```python
from build123d import *

# Parameters (mm, degrees)
SKETCH1_W           = 26.25
SKETCH1_H           = 22
SKETCH1_R           = 3
BOSS_EXTRUDE1_DEPTH = 3
FILLET1_R           = 5
SKETCH2_R           = 1.625
CUT_EXTRUDE1_DEPTH  = 3
SKETCH5_W           = 20
SKETCH5_H           = 3
BOSS_EXTRUDE2_DEPTH = 10
SKETCH6_R           = 1.65
CUT_EXTRUDE4_DEPTH  = 28
CHAMFER1_SIZE       = 10
CHAMFER1_SIZE_2     = 17.320508076
SKETCH9_W           = 20
SKETCH9_H           = 5
CUT_EXTRUDE6_DEPTH  = 3
FILLET3_R           = 5
SKETCH16_W          = 40
SKETCH16_H          = 8
CUT_EXTRUDE11_DEPTH = 10
SKETCH17_R          = 1.25
CUT_EXTRUDE12_DEPTH = 10
SKETCH18_W          = 114.543980026
SKETCH18_H          = 4
CUT_EXTRUDE13_DEPTH = 10
SKETCH3_R           = 1.625
CUT_EXTRUDE14_DEPTH = 10


# Some blends are built 0.0001 mm under size
with BuildPart() as part:
    # Sketch1 → Boss-Extrude1 (new body)
    # profile 1 of 3: a face of its own
    with BuildSketch(Plane(origin=(0, 0, 0), x_dir=(1, 0, 0), z_dir=(0, 1, 0))):
        with Locations((18.375, 0)):
            Rectangle(SKETCH1_W, SKETCH1_H)
        with Locations(Location((20, 0, 0), (0, 0, 270))):
            Circle(SKETCH1_R, mode=Mode.SUBTRACT)
    # profile 2 of 3: a face of its own
    with BuildSketch(Plane(origin=(0, 0, 0), x_dir=(1, 0, 0), z_dir=(0, 1, 0))):
        with Locations((-18.375, 0)):
            Rectangle(SKETCH1_W, SKETCH1_H)
        with Locations(Location((-20, 0, 0), (0, 0, 270))):
            Circle(SKETCH1_R, mode=Mode.SUBTRACT)
    # profile 3 of 3: a face of its own
    with BuildSketch(Plane(origin=(0, 0, 0), x_dir=(1, 0, 0), z_dir=(0, 1, 0))):
        with BuildLine():
            Line((-5.25, -11), (-31.5, -11))
            Line((-31.5, -11), (-50, -11))
            add(Edge.make_bspline(
                [(-50, -11), (-77.2307176, -35.658609428), (-60, -76)],
                knots=[0, 0, 0, 1, 1, 1], degree=2))
            Line((-60, -76), (-22, -76))
            Line((-22, -76), (-22, -51))
            Line((-22, -51), (22, -51))
            Line((22, -51), (22, -76))
            Line((22, -76), (60, -76))
            add(Edge.make_bspline(
                [(50, -11), (77.2307176, -35.658609428), (60, -76)],
                knots=[0, 0, 0, 1, 1, 1], degree=2))
            Line((50, -11), (31.5, -11))
            Line((31.5, -11), (5.25, -11))
            Line((5.25, -11), (-5.25, -11))
        make_face()
    extrude(amount=BOSS_EXTRUDE1_DEPTH)

    # Fillet1
    fillet1_edges = [part.edges().sort_by_distance(p)[0] for p in [
        (60, 1.5, 76),
        (-60, 1.5, 76),
    ]]
    fillet(fillet1_edges, radius=FILLET1_R)

    # Sketch2 → Cut-Extrude1 (cut)
    with BuildSketch(Plane(origin=(0, 3, 0), x_dir=(1, 0, 0), z_dir=(0, 1, 0))):
        with Locations(Location((-60, -56, 0), (0, 0, 270))):
            Circle(SKETCH2_R)
        with Locations(Location((60, -56, 0), (0, 0, 270))):
            Circle(SKETCH2_R)
        with Locations(Location((-45, -17, 0), (0, 0, 270))):
            Circle(SKETCH2_R)
        with Locations(Location((-60, -34, 0), (0, 0, 270))):
            Circle(SKETCH2_R)
        with Locations(Location((60, -34, 0), (0, 0, 270))):
            Circle(SKETCH2_R)
        with Locations(Location((45, -17, 0), (0, 0, 270))):
            Circle(SKETCH2_R)
        with Locations(Location((0, -18, 0), (0, 0, 270))):
            Circle(SKETCH2_R)
        with Locations(Location((0, -36, 0), (0, 0, 270))):
            Circle(SKETCH2_R)
    extrude(amount=-CUT_EXTRUDE1_DEPTH, mode=Mode.SUBTRACT)

    # Sketch5 → Boss-Extrude2 (add)
    with BuildSketch(Plane(origin=(0, 3, 0), x_dir=(1, 0, 0), z_dir=(0, 1, 0))):
        with Locations((0, -49.5)):
            Rectangle(SKETCH5_W, SKETCH5_H)
    extrude(amount=BOSS_EXTRUDE2_DEPTH)

    # Sketch6 → Cut-Extrude4 (cut)
    with BuildSketch(Plane.XY.offset(76)):
        with Locations((0, 5)):
            Circle(SKETCH6_R)
        with Locations((0, 5.5)):
            Circle(SKETCH6_R)
        with Locations((0, 4.5)):
            Circle(SKETCH6_R)
    extrude(amount=-CUT_EXTRUDE4_DEPTH, mode=Mode.SUBTRACT)

    # Chamfer1
    # the kernel refuses this chamfer: 17.320508076, 10 mm, written as the material it adds along each edge
    with BuildSketch(Plane(origin=(-10, 3, 51), x_dir=(-0.9983227437537926, -0.05789386240267139, 0), z_dir=(0, 0, -1))) as chamfer1_piece_1_section:
        Polygon((CHAMFER1_SIZE * 0.998322743754, CHAMFER1_SIZE * 0.0578938624027), (-CHAMFER1_SIZE_2 * 0.0578938624016, CHAMFER1_SIZE_2 * 0.998322743736), (0, 0), align=None)
    chamfer1_piece_1 = extrude(amount=3, mode=Mode.PRIVATE)
    chamfer1_piece_1 = split(chamfer1_piece_1, bisect_by=Plane(origin=(-13.731694811, 13, 49.5), z_dir=(0, -1, 0)), keep=Keep.TOP, mode=Mode.PRIVATE)
    add(chamfer1_piece_1)
    with BuildSketch(Plane(origin=(10, 3, 48), x_dir=(0.9983227437537926, -0.05789386240267137, 0), z_dir=(0, 0, 1))) as chamfer1_piece_2_section:
        Polygon((CHAMFER1_SIZE * 0.998322743754, CHAMFER1_SIZE * 0.0578938624027), (-CHAMFER1_SIZE_2 * 0.0578938624016, CHAMFER1_SIZE_2 * 0.998322743736), (0, 0), align=None)
    chamfer1_piece_2 = extrude(amount=3, mode=Mode.PRIVATE)
    chamfer1_piece_2 = split(chamfer1_piece_2, bisect_by=Plane(origin=(13.731694811, 13, 49.5), z_dir=(0, -1, 0)), keep=Keep.TOP, mode=Mode.PRIVATE)
    add(chamfer1_piece_2)

    # Sketch9 → Cut-Extrude6 (cut)
    with BuildSketch(Plane(origin=(0, 3, 0), x_dir=(1, 0, 0), z_dir=(0, 1, 0))):
        with Locations((0, -45.5)):
            Rectangle(SKETCH9_W, SKETCH9_H)
    extrude(amount=-CUT_EXTRUDE6_DEPTH, mode=Mode.SUBTRACT)

    # Fillet3
    fillet3_edges = [part.edges().sort_by_distance(p)[0] for p in [
        (-10, 1.5, 43),
        (10, 1.5, 43),
    ]]
    fillet(fillet3_edges, radius=FILLET3_R - 0.0001)  # a hair under: the kernel refuses the full size

    # Sketch16 → Cut-Extrude11 (cut)
    with BuildSketch(Plane(origin=(0, 3, 0), x_dir=(1, 0, 0), z_dir=(0, 1, 0))):
        with Locations((0, -26)):
            Rectangle(SKETCH16_W, SKETCH16_H)
    extrude(amount=-CUT_EXTRUDE11_DEPTH, mode=Mode.SUBTRACT)

    # Sketch17 → Cut-Extrude12 (cut)
    with BuildSketch(Plane(origin=(0, 3, 0), x_dir=(1, 0, 0), z_dir=(0, 1, 0))):
        with Locations(Location((-30.5, -17.75, 0), (0, 0, 270))):
            Circle(SKETCH17_R)
        with Locations(Location((-30.5, -38.25, 0), (0, 0, 270))):
            Circle(SKETCH17_R)
        with Locations(Location((30.5, -38.25, 0), (0, 0, 270))):
            Circle(SKETCH17_R)
        with Locations(Location((30.5, -17.75, 0), (0, 0, 270))):
            Circle(SKETCH17_R)
    extrude(amount=-CUT_EXTRUDE12_DEPTH, mode=Mode.SUBTRACT)

    # Sketch18 → Cut-Extrude13 (cut)
    with BuildSketch(Plane(origin=(0, 3, 0), x_dir=(1, 0, 0), z_dir=(0, 1, 0))):
        with Locations((-4.144236525, 9)):
            Rectangle(SKETCH18_W, SKETCH18_H)
    extrude(amount=-CUT_EXTRUDE13_DEPTH, mode=Mode.SUBTRACT)

    # Sketch3 → Cut-Extrude14 (cut)
    with BuildSketch(Plane(origin=(0, 3, 0), x_dir=(1, 0, 0), z_dir=(0, 1, 0))):
        with Locations(Location((-38, -60, 0), (0, 0, 270))):
            Circle(SKETCH3_R)
        with Locations(Location((38, -60, 0), (0, 0, 270))):
            Circle(SKETCH3_R)
    extrude(amount=-CUT_EXTRUDE14_DEPTH, mode=Mode.SUBTRACT)


solid = part.part
```
Verification items for the finished model (mm, model axes). A direction names the side the tool comes from. Give positions to 0.01 mm unless a question says otherwise; leave off trailing zeros. Write each loop counter-clockwise with the first axis right and the second up, starting at its lowest first coordinate (ties: lowest second). Pieces come first, ordered by that corner, then holes. Notation, with made-up numbers: (-17.5, -16) - (37.5, -16) arc R17 cw to (37.5, 13) - close; hole circle Ø9 at (47, 17.25). An arc over 180 degrees is marked (long way). Put each result on its own line as item: value.
Q1. Section check C-C on x = -60. Count the separate pieces of the cut face and the enclosed holes in it, and give its area (3 significant figures).
Result:
separate pieces: 3
enclosed holes: 0
area: 136 mm2
Q2. Section check A-A on z = 0. Record the cut outline in (x, y).
Result:
outline: (-31.5, 0) - (-23, 0) - (-23, 3) - (-31.5, 3) - close; (-17, 0) - (-5.25, 0) - (-5.25, 3) - (-17, 3) - close; (5.25, 0) - (17, 0) - (17, 3) - (5.25, 3) - close; (23, 0) - (31.5, 0) - (31.5, 3) - (23, 3) - close
Q3. Set-up check for faces 1 (the face through (31.5, 1, 2)), 2 (the face through (-5.25, 1, 2)), 3 (the face through (20, 2, 26)): record each of +Z, -Z, +X, -X, +Y, -Y from which the full face is reachable in a straight line by a thin tool's end or side.
Result:
face 1: -Z, +X, +Y, -Y
face 2: -Z, +Y, -Y
face 3: +Y, -Y
Q4. Mould release check, pull along Z, two halves, no side actions. Record for faces 4 (the face through (0, 13, 50)), 5 (the face through (-19, 2, -7)), 6 (the face through (-0.62, 1.52, 19.5)), 7 (the face through (-20, 2, 26)): released by +Z, released by -Z, zero draft, split by the parting line, or undercut.
Result:
face 4: zero draft
face 5: released by -Z
face 6: undercut
face 7: undercut
Q5. Section check B-B on x = 27. Record the cut outline in (y, z).
Result:
outline: (0, -7) - (3, -7) - (3, 76) - (0, 76) - close
Q6. Section check D-D on x = 41.5. Record the cut outline in (y, z).
Result:
outline: (0, 11) - (3, 11) - (3, 76) - (0, 76) - close
Q7. Scan lines: probe 1 along Z at (x, y) = (12, 1.5); probe 2 along Y at (x, z) = (0, 49); probe 3 along X at (y, z) = (2.2, 17.75). Record each from-to range of solid material in increasing order. Write a range as from..to.
Result:
probe 1: -7..22, 30..51
probe 2: 0..2.85, 7.15..13
probe 3: -56.39..-46.44, -43.56..-31.75, -29.25..-1.61, 1.61..29.25, 31.75..43.56, 46.44..56.39
Q8. Depth check by flat-ended pin: P1, Ø4.5, axis at x = 0, y = 5.5, coming from the -Z side; P2, Ø2.5, axis at x = 0, z = 36, coming from the +Y side (1 decimal); P3, Ø0.9, axis at x = -0.5, y = 2, coming from the -Z side; P4, Ø2.5, axis at y = 1.5, z = 3.5, coming from the +X side. Enter the tip coordinate at first touch or a pass-through.
Result:
P1: z = 48
P2: through
P3: z = 11
P4: x = 31.5
